from build123d import *

# Parameters (mm, degrees)
SKETCH1_R           = 50
BOSS_EXTRUDE1_DEPTH = 650
BOSS_EXTRUDE2_DEPTH = 695


with BuildPart() as part:
    # Sketch1 → Boss-Extrude1 (new, symmetric)
    with BuildSketch(Plane.XY):
        Circle(SKETCH1_R)
    extrude(amount=BOSS_EXTRUDE1_DEPTH, both=True)

    # Sketch4 → Boss-Extrude2 (add, symmetric)
    with BuildSketch(Plane.XY):
        with BuildLine():
            Line((-5, 14.142135624), (-5, 18.3))
            Line((-5, 18.3), (5, 18.3))
            Line((5, 18.3), (5, 14.142135624))
            ThreePointArc((5, 14.142135624), (0, -15), (-5, 14.142135624))
        make_face()
    extrude(amount=BOSS_EXTRUDE2_DEPTH, both=True)


solid = part.part
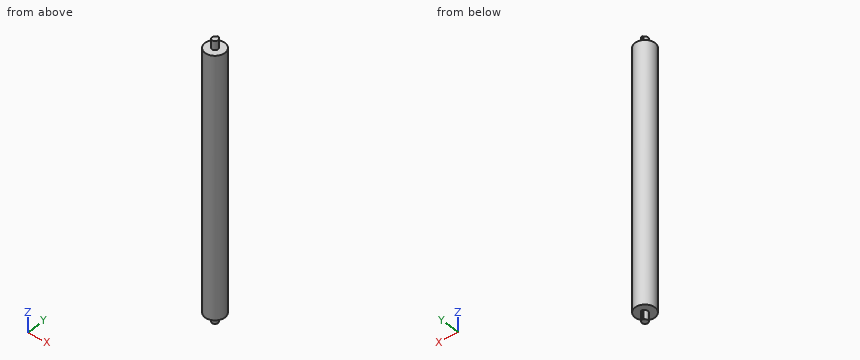
Source: CAD feature listing. Evaluate the final solid. Frame: model axes, mm. Give positions to 0.01 mm unless a question says otherwise; leave off trailing zeros. Write each loop counter-clockwise with the first axis right and the second up, starting at its lowest first coordinate (ties: lowest second). Pieces come first, ordered by that corner, then holes. Notation, with made-up numbers: (-19, -17.5) -> (-13, -17.5) arc R16 cw to (-13, -9.5) -> close; hole circle Ø2 at (60, 14.5). An arc over 180 degrees is marked (long way). Return JSON: item names as keys, results as strings. Group by question number.
1. Pin query (flat end, axial travel): pin 1 Ø1.5 at (x, z) = (0.5, 347) entering from +Y; pin 2 Ø5 at (x, z) = (1.5, -678) entering from +Y; pin 3 Ø4 at (x, z) = (-17, -432) entering from +Y. Return the tip coordinate at first contact, or that it passes through.
2. Section C-C, the plane x = -33. Output: boundary loops of the cut face in (y, z).
3. Section A-A, the plane y = 0. Output: boundary loops of the cut face in (x, z).
4. Section B-B, the plane z = 21. Output: boundary loops of the cut face in (x, y).
5. Material intervals for line 1 (Z direction, x = 38, y = -5.5); line 2 (Y direction, x = -2.5, z = 413); line 3 (X direction, y = -2, z = -177), sorted ascending. Write a range as from..to.
Determined:
{
 "1": {"pin 1": "stops at y = 50", "pin 2": "stops at y = 18.3", "pin 3": "stops at y = 47.7"},
 "2": {"outline": "(-37.56, -650) -> (37.56, -650) -> (37.56, 650) -> (-37.56, 650) -> close"},
 "3": {"outline": "(-50, -650) -> (-15, -650) -> (-15, -695) -> (15, -695) -> (15, -650) -> (50, -650) -> (50, 650) -> (15, 650) -> (15, 695) -> (-15, 695) -> (-15, 650) -> (-50, 650) -> close"},
 "4": {"outline": "circle Ø100 at (0, 0)"},
 "5": {"line 1": "z = -650..650", "line 2": "y = -49.94..49.94", "line 3": "x = -49.96..49.96"}
}
